Work out the finished part from the listing and answer in its coordinate system (mm). A direction names the side the tool comes from. Round coordinates to 2 decimals unless told otherwise and drop trailing zeros. Write each loop counter-clockwise with the first axis right and the second up, starting at its lowest first coordinate (ties: lowest second). Pieces come first, ordered by that corner, then holes.
1. Find section A-A (z = 0). Write down the section's boundary in (x, y).
2. Determine the mould class of faces 6 (the face through (7.46, -9.76, 2.17)), 7 (the face through (-21.035, -21.238, 21.188)), 8 (the face through (0, -7, -13)) for opening direction Y: pulls with the +Y half, pulls with the -Y half, needs draft (parallel to the pull), parting line crosses it, or undercut.
3. Straight lines are drawn through the part: probe 1 along Z at (x, y) = (2, -7) (3 decimals); probe 2 along Y at (x, z) = (2, 0); probe 3 along X at (y, z) = (-9, 5). For each, find the intervals that lie inside material, in ascending order.
4. Find section B-B (y = 15). Write down the section's boundary in (x, z), and give its area (3 significant figures).
5. Find section D-D (x = 8.5). Write down the section's boundary in (y, z), and give its area (3 significant figures).
6. Find section C-C (x = 3). Write down the section's boundary in (y, z), and give its area (3 significant figures).
7. Flat-ended cylindrical pins translate along their axes: pin 1 Ø2.5 at (y, z) = (15, 0.5) entering from +X; pin 2 Ø10 at (x, y) = (-12, -7) entering from +Z; pin 3 Ø5 at (x, z) = (11.5, 8) entering from -Y. Find the tip coordinate at first contact, or state that the pin passes through.
8. A tool of negligible diameter and unlimited length cuts with its end or side. For faces 1 (the face through (0, -14, 15)), 2 (the face through (-23.48, -18.22, 17.76)), 3 (the face through (20, 2, 0)), 4 (the face through (25, 0, 0)), 5 (the face through (2.54, 16.01, 1.11)), from which of +Z, -Z, +X, -X, +Y, -Y can it reach the whole face along a straight path? Write none if from no direction.
```python
from build123d import *
from build123d.topology import SkipClean

# Parameters (mm, degrees)
SKETCH_1_R                       = 20
EXTRUDE_1_DEPTH                  = 5
SKETCH_2_R                       = 10
EXTRUDE_2_DEPTH                  = 5
SKETCH_3_R                       = 1.5
CUT_EXTRUDE_1_DEPTH              = 5
SKETCH_4_R                       = 3
EXTRUDE_3_DEPTH                  = 5
EXTRUDE_4_DEPTH                  = 10
EXTRUDE_START                    = 26
SKETCH_6_R                       = 20
EXTRUDE_5_DEPTH                  = 26
SKETCH_8_R                       = 2.5
EXTRUDE_6_DEPTH                  = 10
EXTRUDE_6_DIRECTION_2_REACH      = 56.84
EXTRUDE_6_DIRECTION_2_END_RADIUS = 20
SKETCH_9_W                       = 26
SKETCH_9_H                       = 8
EXTRUDE_7_DEPTH                  = 1
EXTRUDE_7_DIRECTION_2_REACH      = 56.84
EXTRUDE_7_DIRECTION_2_END_RADIUS = 20


with BuildPart() as part:
    # Эскиз1 → Бобышка-Вытянуть1 (new body)
    with BuildSketch(Plane(origin=(0, 0, 0), x_dir=(0, 0, -1), z_dir=(1, 0, 0))):
        Circle(SKETCH_1_R)
    extrude(amount=EXTRUDE_1_DEPTH)

    # Эскиз2 → Бобышка-Вытянуть2 (add)
    with BuildSketch(Plane(origin=(5, 0, 0), x_dir=(0, 0, -1), z_dir=(1, 0, 0))):
        Circle(SKETCH_2_R)
    extrude(amount=EXTRUDE_2_DEPTH)

    # Эскиз3 → Вырез-Вытянуть1 (cut)
    with BuildSketch(Plane(origin=(5, 0, 0), x_dir=(0, 0, -1), z_dir=(1, 0, 0))):
        with Locations((0, 15)):
            Circle(SKETCH_3_R)
        with Locations((12.990381057, -7.5)):
            Circle(SKETCH_3_R)
        with Locations((-12.990381057, -7.5)):
            Circle(SKETCH_3_R)
    extrude(amount=-CUT_EXTRUDE_1_DEPTH, mode=Mode.SUBTRACT)

    # Эскиз4 → Бобышка-Вытянуть3 (add)
    with BuildSketch(Plane(origin=(10, 0, 0), x_dir=(0, 0, -1), z_dir=(1, 0, 0))):
        Circle(SKETCH_4_R)
    extrude(amount=EXTRUDE_3_DEPTH)

    # Эскиз5 → Бобышка-Вытянуть4 (add)
    with BuildSketch(Plane(origin=(15, 0, 0), x_dir=(0, 0, -1), z_dir=(1, 0, 0))):
        with BuildLine():
            Line((-2.236067977, 2), (2.236067977, 2))
            ThreePointArc((2.236067977, 2), (0, -3), (-2.236067977, 2))
        make_face()
    extrude(amount=EXTRUDE_4_DEPTH)

    # Эскиз6 → Бобышка-Вытянуть5 (add)
    with BuildSketch(Plane.ZY.offset(EXTRUDE_START)):
        Circle(SKETCH_6_R)
    extrude(amount=-EXTRUDE_5_DEPTH)

    # Эскиз8 → Бобышка-Вытянуть6 (add)
    with BuildSketch(Plane(origin=(0, -14.142135624, 14.142135624), x_dir=(-1, 0, 0), z_dir=(0, -0.7071067811865511, 0.707106781186544))):
        with Locations(Location((21, 0, 0), (0, 0, 270))):
            Circle(SKETCH_8_R)
    extrude(amount=EXTRUDE_6_DEPTH)

    # Бобышка-Вытянуть6 direction 2: up to this cylinder (the profile starts outside it)
    with SkipClean():  # the faces are left unmerged after this step: merging them gives an invalid solid
        extrude_6_direction_2_end = Plane(origin=(-21, 0, 0), z_dir=(-1, 0, 0)) * Cylinder(EXTRUDE_6_DIRECTION_2_END_RADIUS, 154.68, mode=Mode.PRIVATE)
        # Эскиз8 → Бобышка-Вытянуть6 direction 2 (add, up to the surface)
        with BuildSketch(Plane(origin=(0, -14.142135624, 14.142135624), x_dir=(-1, 0, 0), z_dir=(0, -0.7071067811865511, 0.707106781186544)), mode=Mode.PRIVATE) as extrude_6_direction_2_sk1:
            with Locations(Location((21, 0, 0), (0, 0, 270))):
                Circle(SKETCH_8_R)
        extrude_6_direction_2_tool1 = extrude(extrude_6_direction_2_sk1.sketch, amount=-EXTRUDE_6_DIRECTION_2_REACH, mode=Mode.PRIVATE) - extrude_6_direction_2_end
        add(extrude_6_direction_2_tool1.solids().sort_by_distance((-21, -14.142136, 14.142136))[0])
        add(extrude_6_direction_2_tool1.solids().sort_by_distance((-21, -14.142136, 14.142136))[1])

    # Эскиз9 → Бобышка-Вытянуть7 (add)
    with SkipClean():  # the faces are left unmerged after this step: merging them gives an invalid solid
        with BuildSketch(Plane(origin=(0, -14.142135624, 14.142135624), x_dir=(-1, 0, 0), z_dir=(0, -0.7071067811865511, 0.707106781186544))):
            with Locations((13, 0)):
                Rectangle(SKETCH_9_W, SKETCH_9_H)
        extrude(amount=EXTRUDE_7_DEPTH)

    # Бобышка-Вытянуть7 direction 2: up to this cylinder (the profile starts outside it)
    with SkipClean():  # the faces are left unmerged after this step: merging them gives an invalid solid
        extrude_7_direction_2_end = Plane(origin=(-13, 0, 0), z_dir=(-1, 0, 0)) * Cylinder(EXTRUDE_7_DIRECTION_2_END_RADIUS, 154.68, mode=Mode.PRIVATE)
        # Эскиз9 → Бобышка-Вытянуть7 direction 2 (add, up to the surface)
        with BuildSketch(Plane(origin=(0, -14.142135624, 14.142135624), x_dir=(-1, 0, 0), z_dir=(0, -0.7071067811865511, 0.707106781186544)), mode=Mode.PRIVATE) as extrude_7_direction_2_sk1:
            with Locations((13, 0)):
                Rectangle(SKETCH_9_W, SKETCH_9_H)
        extrude_7_direction_2_tool1 = extrude(extrude_7_direction_2_sk1.sketch, amount=-EXTRUDE_7_DIRECTION_2_REACH, mode=Mode.PRIVATE) - extrude_7_direction_2_end
        add(extrude_7_direction_2_tool1.solids().sort_by_distance((-13, -14.142136, 14.142136))[0])
        add(extrude_7_direction_2_tool1.solids().sort_by_distance((-13, -14.142136, 14.142136))[1])


solid = part.part
```
Worked answers:
1. outline: (-26, -20) - (5, -20) - (5, -10) - (10, -10) - (10, -3) - (25, -3) - (25, 2) - (15, 2) - (15, 3) - (10, 3) - (10, 10) - (5, 10) - (5, 13.5) - (0, 13.5) - (0, 16.5) - (5, 16.5) - (5, 20) - (-26, 20) - close
2. face 6: parting line crosses it
2. face 7: pulls with the -Y half
2. face 8: undercut
3. probe 1: z = -18.735 to -14.405, -11.576 to 11.576, 14.405 to 18.735
3. probe 2: y = -20 to 13.5, 16.5 to 20
3. probe 3: x = -26 to 5
4. outline: (-26, -13.23) - (5, -13.23) - (5, -1.5) - (0, -1.5) - (0, 1.5) - (5, 1.5) - (5, 13.23) - (-26, 13.23) - close
4. area: 805 mm2
5. outline: circle Ø20 at (0, 0)
5. area: 314 mm2
6. outline: circle Ø40 at (0, 0); hole circle Ø3 at (-7.5, -12.99); hole circle Ø3 at (-7.5, 12.99); hole circle Ø3 at (15, 0)
6. area: 1,240 mm2
7. pin 1: stops at x = 5
7. pin 2: stops at z = 19.9
7. pin 3: stops at y = -8
8. face 1: +Z, +X, -Y
8. face 2: none
8. face 3: +Z, -Z, +X, +Y
8. face 4: +Z, -Z, +X, +Y, -Y
8. face 5: +X
